Could you check a few things on this model? Use its own coordinates, in mm. A direction names the side the tool comes from. Round coordinates to 2 decimals unless told otherwise and drop trailing zeros. Write each loop counter-clockwise with the first axis right and the second up, starting at its lowest first coordinate (ties: lowest second). Pieces come first, ordered by that corner, then holes. Notation, with made-up numbers: M 12.5,4.5 L 64.5,4.5 A8 cw 64.5,9.5 Z; hole C 76,68.5 d7. An arc over 180 degrees is marked long. One line per item, written item: value. Start each with the question number.
(1) Thinking about a two-plate mould opening in X: for faces 1 (the face through (1.325, -1.493, -1.277)), 2 (the face through (-1, 62, 1)), 3 (the face through (-1, 57, -1)), which applies, released by +X, released by -X, zero draft, split by the parting line, or undercut?
(2) I want a section at C-C on y = 27. Please give me the cut outline in (x, z), and give its area (3 significant figures).
(3) Which directions (+Z, -Z, +X, -X, +Y, -Y) give clear straight access to the entire face, cutting with the end or side of a thin tool? Please do faces 4 (the face through (1, -1, 0)), 5 (the face through (-1.4, 59.5, -1.4)), 6 (the face through (-2.308, 30.566, 0.858)).
(4) If I drill on L1, parallel to Y at x = -0.65, z = 1.4; L2, parallel to Z at x = -0.65, y = 51; L3, parallel to Y at x = -0.25, z = -0.1, over which ranges is the centre line in solid material (lowest first)?
(5) I want a section at A-A on z = -1.15. Please give me the cut outline in (x, y), and give its area (3 significant figures).
(6) I'm going to push flat-ended pins straight in: pin 1 Ø2 at (x, y) = (-1, 15) entering from -Z; pin 2 Ø1.2 at (x, z) = (0, -0.5) entering from +Y. Where does each tip first touch, or does it pass through?
(7) I want a section at B-B on x = -0.65. Please give me the cut outline in (y, z).
```python
from build123d import *

# Parameters (mm, degrees)
SKETCH1_R           = 2.25
BOSS_EXTRUDE1_DEPTH = 62
SKETCH1_3_R         = 1
BOSS_EXTRUDE2_DEPTH = 1
SKETCH5_R           = 1.25
BOSS_EXTRUDE3_DEPTH = 1
SKETCH6_R           = 2
BOSS_EXTRUDE4_DEPTH = 1
SKETCH12_R          = 1.25
CUT_EXTRUDE1_DEPTH  = 5


with BuildPart() as part:
    # Sketch1 → Boss-Extrude1 (new body)
    with BuildSketch(Plane(origin=(0, 0, 0), x_dir=(1, 0, 0), z_dir=(0, 1, 0))):
        with Locations((-0.522013312, 0.511138034)):
            Circle(SKETCH1_R)
    extrude(amount=BOSS_EXTRUDE1_DEPTH)

    # Sketch1<3> → Boss-Extrude2 (add)
    with BuildSketch(Plane(origin=(0, 0, 0), x_dir=(1, 0, 0), z_dir=(0, 1, 0))):
        with Locations((-0.522013312, 0.511138034)):
            Circle(SKETCH1_3_R)
    extrude(amount=BOSS_EXTRUDE2_DEPTH)

    # Sketch5 → Boss-Extrude3 (add)
    with BuildSketch(Plane.XZ):
        with Locations((-0.522013312, -0.511138034)):
            Circle(SKETCH5_R)
    extrude(amount=BOSS_EXTRUDE3_DEPTH)

    # Sketch6 → Boss-Extrude4 (add)
    with BuildSketch(Plane.XZ.offset(1)):
        with Locations((-0.522013312, -0.511138034)):
            Circle(SKETCH6_R)
    extrude(amount=BOSS_EXTRUDE4_DEPTH)

    # Sketch12 → Cut-Extrude1 (cut)
    with BuildSketch(Plane(origin=(0, 62, 0), x_dir=(1, 0, 0), z_dir=(0, 1, 0))):
        with Locations((-0.522013312, 0.511138034)):
            Circle(SKETCH12_R)
    extrude(amount=-CUT_EXTRUDE1_DEPTH, mode=Mode.SUBTRACT)


solid = part.part
```
Found:
1. face 1: split by the parting line
1. face 2: zero draft
1. face 3: undercut
2. outline: C -0.52,-0.51 d4.5
2. area: 15.9 mm²
3. face 4: none
3. face 5: +Y
3. face 6: +Y, -Y
4. L1: y = -2 to -1, 0 to 62
4. L2: z = -2.76 to 1.74
4. L3: y = -2 to 57
5. outline: M -2.68,0 L -1.6,0 L -1.6,-1 L -2.42,-1 L -2.42,-2 L 1.37,-2 L 1.37,-1 L 0.55,-1 L 0.55,0 L 1.64,0 L 1.64,62 L 0.55,62 L 0.55,57 L -1.6,57 L -1.6,62 L -2.68,62 Z
5. area: 263 mm²
6. pin 1: stops at z = -2.76
6. pin 2: stops at y = 57
7. outline: M -2,-2.51 L -1,-2.51 L -1,-1.75 L 0,-1.75 L 0,-2.76 L 62,-2.76 L 62,-1.75 L 57,-1.75 L 57,0.73 L 62,0.73 L 62,1.74 L 0,1.74 L 0,0.73 L -1,0.73 L -1,1.48 L -2,1.48 Z
